The model under review builds one solid part; all positions refer to its coordinate system, in mm. A direction names the side the tool comes from. Round coordinates to 2 decimals unless told otherwise and drop trailing zeros. Write each loop counter-clockwise with the first axis right and the second up, starting at its lowest first coordinate (ties: lowest second). Pieces come first, ordered by that corner, then holes. Notation, with made-up numbers: (11.25, 19) -> (47.25, 19) arc R21 ccw to (47.25, 49) -> close; hole circle Ø2 at (20, 66). An arc over 180 degrees is marked (long way). Answer as a JSON object with one key per item and string values. Group by question number.
1) Mouldability with a two-part tool opening along Y and no side actions: class faces 4 (the cylindrical face through (-1.216, 1.115, 3.65)), 5 (the cylindrical face through (-0.867, -3.905, 4.817)), 6 (the flat face through (4, -2, 0)) as pulls with the +Y half, pulls with the -Y half, needs draft (parallel to the pull), parting line crosses it, or undercut.
2) Insertion check: pin 1 Ø1 at (x, y) = (-4, 2.5) entering from +Z; pin 2 Ø10 at (y, z) = (2.5, -7) entering from -X; pin 3 Ø2 at (y, z) = (0, -21.5) entering from +X. Each pin has a flat end and moves straight along its axis. Give the tip position at first contact, or say it passes through.
3) We need section D-D, the plane y = -7.5. Write out the cut boundary in (x, z), then the cut area to 3 significant figures.
4) To check wall thickness, follow probe 1 along Y at (x, z) = (0, 3); probe 2 along Z at (x, y) = (5, 5.5); probe 3 along Y at (x, z) = (0, 2.25). State the ranges of each line that lie inside material, in increasing order. Write a range as [from, to].
5) We need section A-A, the plane y = 0. Write out the cut boundary in (x, z).
6) We need section C-C, the plane z = -6. Write out the cut boundary in (x, y), then the cut area to 3 significant figures.
7) Machinability: for faces 1 (the cylindrical face through (-0.867, 3.905, -15.21)), 2 (the cylindrical face through (4.57, 7.167, 1.232)), 3 (the flat face through (0, 0, 0)), which of the approach directions +Z, -Z, +X, -X, +Y, -Y give a long, thin tool a straight path to every point of the face, cutting with its end or side? Answer none if there is none.
from build123d import *

# Parameters (mm, degrees)
SKETCH_1_R          = 8.5
EXTRUDE_1_DEPTH     = 2.5
SKETCH_2_R          = 4
EXTRUDE_2_DEPTH     = 4.7
SKETCH_3_R          = 1.65
CUT_EXTRUDE_1_DEPTH = 12
EXTRUDE_START       = 30
SKETCH_4_R          = 4
EXTRUDE_3_DEPTH     = 30


with BuildPart() as part:
    # Эскиз1 → Бобышка-Вытянуть1 (new body)
    with BuildSketch(Plane.XY):
        Circle(SKETCH_1_R)
    extrude(amount=EXTRUDE_1_DEPTH)

    # Эскиз2 → Бобышка-Вытянуть2 (add)
    with BuildSketch(Plane.XY.offset(2.5)):
        Circle(SKETCH_2_R)
    extrude(amount=EXTRUDE_2_DEPTH)

    # Эскиз3 → Вырез-Вытянуть1 (cut)
    with BuildSketch(Plane.XY.offset(7.2)):
        Circle(SKETCH_3_R)
    extrude(amount=-CUT_EXTRUDE_1_DEPTH, mode=Mode.SUBTRACT)

    # Эскиз4 → Бобышка-Вытянуть3 (add)
    with BuildSketch(Plane(origin=(0, 0, 0), x_dir=(-1, 0, 0), z_dir=(0, 0, -1)).offset(EXTRUDE_START)):
        with Locations(Location((0, 0, 0), (0, 0, 180))):
            Circle(SKETCH_4_R)
    extrude(amount=-EXTRUDE_3_DEPTH)


solid = part.part
Here are the results:
{
 "1": {"face 4": "undercut", "face 5": "parting line crosses it", "face 6": "needs draft"},
 "2": {"pin 1": "stops at z = 2.5", "pin 2": "stops at x = -4", "pin 3": "stops at x = 4"},
 "3": {"outline": "(-4, 0) -> (4, 0) -> (4, 2.5) -> (-4, 2.5) -> close", "area": "20.0 mm^2"},
 "4": {"probe 1": "y = [-4, -1.65], [1.65, 4]", "probe 2": "z = [0, 2.5]", "probe 3": "y = [-8.5, -1.65], [1.65, 8.5]"},
 "5": {"outline": "(-8.5, 0) -> (-4, 0) -> (-4, -30) -> (4, -30) -> (4, 0) -> (8.5, 0) -> (8.5, 2.5) -> (4, 2.5) -> (4, 7.2) -> (1.65, 7.2) -> (1.65, 0) -> (-1.65, 0) -> (-1.65, 7.2) -> (-4, 7.2) -> (-4, 2.5) -> (-8.5, 2.5) -> close"},
 "6": {"outline": "circle Ø8 at (0, 0)", "area": "50.3 mm^2"},
 "7": {"face 1": "-Z", "face 2": "+Z, -Z", "face 3": "+Z"}
}
